Design review of the part shown in the three views and the two pictorial views. Dimensions are in mm from the part's minimum x, y and z. A direction names the side the tool comes from. Round coordinates to 2 decimals unless told otherwise and drop trailing zeros. Order: outer loops, then holes, each group sorted by start corner. A loop starts at its lowest first (then second) coordinate and runs counter-clockwise, first axis right, second up. Notation, with made-up numbers: M 85.25,46 L 109.25,46 A32 cw 109.25,79 Z; hole C 69,-8.75 d4. An arc over 180 degrees is marked long. Use a Markdown table: item, result. Add a question column.
(1) Take a section at D-D (z = 53.5). Write out the cut boundary in (x, y), then the cut area to 3 significant figures.
(2) Take a section at C-C (x = 19). Write out the cut boundary in (y, z), then the cut area to 3 significant figures.
(3) Take a section at B-B (y = 105). Write out the cut boundary in (x, z), then the cut area to 3 significant figures.
(4) Machinability: for the marked faces 1 and 2, which of the approach directions +Z, -Z, +X, -X, +Y, -Y give a long, thin tool a straight path to every point of the face, cutting with its end or side? Answer none if there is none.
(5) Take a section at A-A (x = 10). Write out the cut boundary in (y, z), then the cut area to 4 significant figures.
(6) To check wall thickness, follow probe 1 along X at (y, z) = (105, 1.9); probe 2 along Y at (x, z) = (50, 1); probe 3 along Y at (x, z) = (18, 16.5). State the ranges of each line that lie inside material, in increasing order. Write a range as from..to.
(7) For pin 1 (8 mm diameter, centred on x = 53, y = 106, fed in from +Z); pin 2 (3 mm diameter, centred on x = 35.5, y = 5, fed in from -Z); pin 3 (1.8 mm diameter, centred on x = 10, y = 105, fed in from +Z); pin 4 (5 mm diameter, centred on y = 104.5, z = 36.5, fed in from -X), all flat-tipped, find the tip position at first contact; note any pin that passes through.
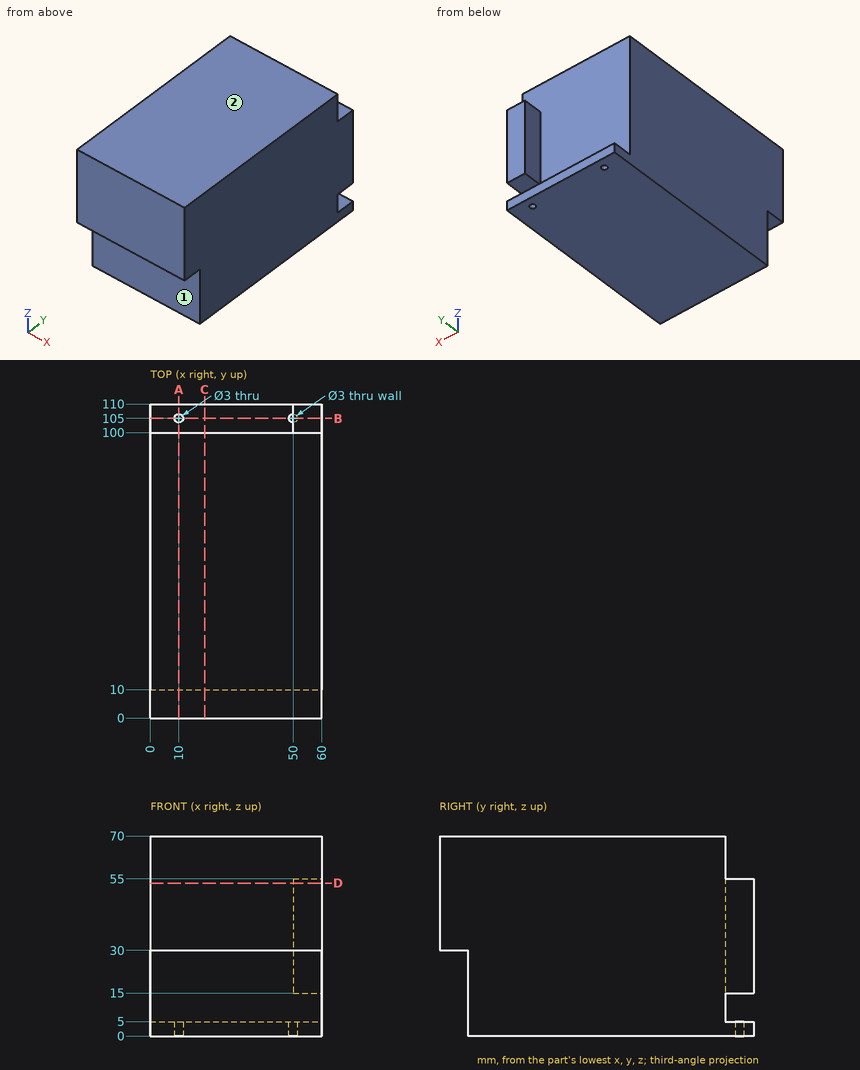
Verdict:
| question | item | result |
|---|---|---|
| 1 | outline | M 0,0 L 60,0 L 60,110 L 50,110 L 50,100 L 0,100 Z |
| 1 | area | 6,100 mm^2 |
| 2 | outline | M 0,30 L 10,30 L 10,0 L 110,0 L 110,5 L 100,5 L 100,70 L 0,70 Z |
| 2 | area | 6,750 mm^2 |
| 3 | outline | M 0,0 L 8.5,0 L 8.5,5 L 0,5 Z; M 11.5,0 L 48.5,0 L 48.5,5 L 11.5,5 Z; M 50,15 L 60,15 L 60,55 L 50,55 Z; M 51.5,0 L 60,0 L 60,5 L 51.5,5 Z |
| 3 | area | 670 mm^2 |
| 4 | face 1 | -Z, +X, -X, -Y |
| 4 | face 2 | +Z, +X, -X, +Y, -Y |
| 5 | outline | M 0,30 L 10,30 L 10,0 L 103.5,0 L 103.5,5 L 100,5 L 100,70 L 0,70 Z; M 106.5,0 L 110,0 L 110,5 L 106.5,5 Z |
| 5 | area | 6,735 mm^2 |
| 6 | probe 1 | x = 0..8.5, 11.5..48.5, 51.5..60 |
| 6 | probe 2 | y = 10..103.5, 106.5..110 |
| 6 | probe 3 | y = 10..100 |
| 7 | pin 1 | stops at z = 55 |
| 7 | pin 2 | stops at z = 30 |
| 7 | pin 3 | passes through |
| 7 | pin 4 | stops at x = 50 |
